Read the model definition and answer for the solid it produces. Units are mm, in the model's axes. A direction names the side the tool comes from. Give positions to 0.01 mm unless a question says otherwise; leave off trailing zeros. Order: outer loops, then holes, each group sorted by start corner. A loop starts at its lowest first (then second) coordinate and runs counter-clockwise, first axis right, second up. Notation, with made-up numbers: (18, 39.25) - (31, 39.25) arc R15 cw to (31, 52.25) - close; hole circle Ø2 at (15.5, -23). An arc over 180 degrees is marked (long way). Return JSON: item names as keys, results as strings.
```python
from build123d import *

# Parameters (mm, degrees)
BOSS_EXTRUDE1_DEPTH = 12.7
CUT_EXTRUDE2_DEPTH  = 4.5
CUT_EXTRUDE3_DEPTH  = 11.2
BOSS_EXTRUDE2_START = -7.7
SKETCH2_5_R         = 1.6
BOSS_EXTRUDE2_DEPTH = 9.1
SKETCH2_6_R         = 1.8
CUT_EXTRUDE4_DEPTH  = 11.2
SKETCH2_7_R         = 1.6
BOSS_EXTRUDE3_DEPTH = 1.4
SKETCH2_8_W         = 36
SKETCH2_8_H         = 0.65
CUT_EXTRUDE5_DEPTH  = 4
CUT_EXTRUDE6_DEPTH  = 3
SKETCH4_W           = 1.5
SKETCH4_H           = 22
CUT_EXTRUDE7_DEPTH  = 3
SKETCH6_W           = 2.1
SKETCH6_H           = 4.185
BOSS_EXTRUDE4_DEPTH = 1
CUT_EXTRUDE9_START  = -10.2
CUT_EXTRUDE9_DEPTH  = 4.5
FILLET3_R           = 1.5
FILLET2_R           = 0.25


with BuildPart() as part:
    # Sketch1 → Boss-Extrude1 (new body)
    with BuildSketch(Plane(origin=(0, 0, 0), x_dir=(1, 0, 0), z_dir=(0, 1, 0))):
        Polygon((-28.77817965, 9.54419618), (-24.27817965, 9.54419618), (-24.27817965, 17.54419618), (-21.57817965, 17.54419618), (-21.57817965, 9.54419618), (-18.57817965, 9.54419618), (-18.57817965, -18.45580382), (-21.07817965, -18.45580382), (-21.07817965, -4.45580382), (-28.77817965, -4.45580382), align=None)
    extrude(amount=BOSS_EXTRUDE1_DEPTH)

    # Sketch2 → Cut-Extrude2 (cut)
    with BuildSketch(Plane.ZY.offset(28.77817965)):
        Polygon((-9.54419618, 3.548072024), (-9.54419618, 0), (-3.657330191, 0), align=None)
    extrude(amount=-CUT_EXTRUDE2_DEPTH, mode=Mode.SUBTRACT)

    # Sketch2<4> → Cut-Extrude3 (cut, through all)
    with BuildSketch(Plane.ZY.offset(28.77817965)):
        Polygon((12.124702683, 0), (18.45580382, 0), (18.45580382, 9.2), align=None)
    extrude(amount=-CUT_EXTRUDE3_DEPTH, mode=Mode.SUBTRACT)

    # Sketch2<5> → Boss-Extrude2 (add)
    with BuildSketch(Plane.ZY.offset(28.77817965).offset(BOSS_EXTRUDE2_START)):
        with Locations((15.20580382, 9.2)):
            Circle(SKETCH2_5_R)
    extrude(amount=BOSS_EXTRUDE2_DEPTH)

    # Sketch2<6> → Cut-Extrude4 (cut, through all)
    with BuildSketch(Plane.ZY.offset(28.77817965)):
        with Locations((-13.54419618, 9.2)):
            Circle(SKETCH2_6_R)
    extrude(amount=-CUT_EXTRUDE4_DEPTH, mode=Mode.SUBTRACT)

    # Sketch2<7> → Boss-Extrude3 (add)
    with BuildSketch(Plane.ZY.offset(28.77817965)):
        with Locations((-6.29419618, 9.2)):
            Circle(SKETCH2_7_R)
    extrude(amount=BOSS_EXTRUDE3_DEPTH)

    # Sketch2<8> → Cut-Extrude5 (cut)
    with BuildSketch(Plane.ZY.offset(28.77817965)):
        with Locations((0.45580382, 11.625)):
            Rectangle(SKETCH2_8_W, SKETCH2_8_H)
    extrude(amount=-CUT_EXTRUDE5_DEPTH, mode=Mode.SUBTRACT)

    # Sketch3 → Cut-Extrude6 (cut)
    with BuildSketch(Plane(origin=(-18.57817965, 0, 0), x_dir=(0, 0, -1), z_dir=(1, 0, 0))):
        Polygon((9.54419618, 0), (9.54419618, 9.2), (-0.27080382, 0), align=None)
        Polygon((-12.124702683, 0), (-18.45580382, 9.2), (-18.45580382, 0), align=None)
        Polygon((-8.64080382, 0), (-18.45580382, 9.2), (-12.124702683, 0), align=None)
    extrude(amount=-CUT_EXTRUDE6_DEPTH, mode=Mode.SUBTRACT)

    # Sketch4 → Cut-Extrude7 (cut)
    with BuildSketch(Plane.XZ):
        with Locations((-22.92817965, -6.54419618)):
            Rectangle(SKETCH4_W, SKETCH4_H)
    extrude(amount=-CUT_EXTRUDE7_DEPTH, mode=Mode.SUBTRACT)

    # Sketch6 → Boss-Extrude4 (add)
    with BuildSketch(Plane(origin=(0, 0, 0), x_dir=(-1, 0, 0), z_dir=(0, -1, 0))):
        with Locations((22.62817965, -2.36330382)):
            Rectangle(SKETCH6_W, SKETCH6_H)
    extrude(amount=-BOSS_EXTRUDE4_DEPTH)

    # Sketch3<3> → Cut-Extrude9 (cut)
    with BuildSketch(Plane(origin=(-18.57817965, 0, 0), x_dir=(0, 0, -1), z_dir=(1, 0, 0)).offset(CUT_EXTRUDE9_START)):
        Polygon((9.54419618, 0), (9.54419618, 9.2), (-0.27080382, 0), align=None)
    extrude(amount=CUT_EXTRUDE9_DEPTH, mode=Mode.SUBTRACT)

    # Fillet3
    fillet3_edges = [part.edges().sort_by_distance(p)[0] for p in [
        (-18.57817965, 0, 4.45580382),
        (-18.57817965, 10.95, 18.45580382),
        (-18.57817965, 4.6, 13.54830382),
        (-18.57817965, 4.6, -4.63669618),
        (-18.57817965, 10.95, -9.54419618),
        (-18.57817965, 12.7, 4.45580382),
        (-24.92817965, 12.7, 4.45580382),
        (-19.82817965, 0, 8.64080382),
        (-19.82817965, 9.2, 18.45580382),
        (-19.82817965, 12.7, 18.45580382),
        (-26.52817965, 0, 0.27080382),
        (-20.07817965, 0, 0.27080382),
        (-20.07817965, 9.2, -9.54419618),
        (-20.07817965, 12.7, -9.54419618),
        (-26.52817965, 9.2, -9.54419618),
        (-26.52817965, 12.7, -9.54419618),
        (-21.87817965, 0, -17.54419618),
        (-23.97817965, 0, -17.54419618),
        (-22.92817965, 12.7, -17.54419618),
    ]]
    fillet(fillet3_edges, radius=FILLET3_R)

    # Fillet2
    fillet2_edges = [part.edges().sort_by_distance(p)[0] for p in [
        (-22.17817965, 3, -6.54419618),
        (-22.17817965, 2, 4.45580382),
        (-22.92817965, 3, -17.54419618),
        (-22.17817965, 2.25, -17.54419618),
        (-23.67817965, 3, -6.54419618),
        (-23.67817965, 2.25, -17.54419618),
        (-22.92817965, 3, 4.45580382),
        (-23.67817965, 2, 4.45580382),
        (-23.67817965, 0, -7.88669618),
        (-22.17817965, 0, -7.88669618),
        (-22.17817965, 0.439339828, -17.104856352),
        (-23.67817965, 0.439339828, -17.104856352),
    ]]
    fillet(fillet2_edges, radius=FILLET2_R)


solid = part.part
```
Q1. Given pin 1 (0.8 mm diameter, centred on y = 12, z = -1.5, fed in from -X); pin 2 (1.1 mm diameter, centred on x = -23.5, y = 0.5, fed in from -Z); pin 3 (0.7 mm diameter, centred on x = -27.5, y = 11, fed in from -Z), each flat-ended and moving along its own axis, determine where each tip first touches the part or whether it passes through.
Values:
{"pin 1": "stops at x = -28.78", "pin 2": "stops at z = -17.42", "pin 3": "stops at z = -9.54"}
Q2. Consider L1, parallel to X at y = 2, z = -4; L2, parallel to X at y = 10.75, z = 4; L3, parallel to X at y = 8.75, z = 12.5. Determine where each line is inside the solid, lowest interval first.
Values:
{"L1": "x = -24.28 to -23.68, -22.18 to -21.58", "L2": "x = -28.78 to -18.58", "L3": "x = -21.08 to -18.58"}
Q3. For faces 1 (the flat face through (-22.9, 0.5, 0.271)), 2 (the flat face through (-20.82, 4.64, -4.68)), 3 (the flat face through (-21, 11, -9.544)), 4 (the flat face through (-25, 6, 4.456)), 5 (the flat face through (-27, 11, -9.544)), determine the directions among +Z, -Z, +X, -X, +Y, -Y from which every point of the face is accessible in a straight line to the end or side of a thin tool.
Values:
{"face 1": "-Z, -Y", "face 2": "-Z, +X, -Y", "face 3": "-Z, +X, +Y, -Y", "face 4": "-X, +Y, -Y", "face 5": "-Z, -X, +Y, -Y"}
Q4. A cutting plane is placed at A-A (x = -23). Write down the section's boundary in (y, z), and give its area (3 significant figures).
Values:
{"outline": "(0, 0.27) - (1, 0.27) - (1, 4.46) - (0, 4.46) - close; (3, -17.29) arc R0.25 ccw to (3.25, -17.54) - (11.2, -17.54) arc R1.5 ccw to (12.7, -16.04) - (12.7, 2.96) arc R1.5 ccw to (11.2, 4.46) - (3.25, 4.46) arc R0.25 ccw to (3, 4.21) - close; circle Ø3.2 at (9.2, 15.21); hole circle Ø3.6 at (9.2, -13.54)", "area": "214 mm²"}
Q5. A cutting plane is placed at C-C (x = -19.5). Write down the section's boundary in (y, z), and give its area (3 significant figures).
Values:
{"outline": "(0.12, 0.86) arc R1.38 ccw to (0.49, -0.08) - (8.84, -8.99) arc R1.38 ccw to (9.85, -9.43) - (11.2, -9.43) arc R1.38 ccw to (12.58, -8.04) - (12.58, 16.96) arc R1.38 ccw to (11.2, 18.34) - (9.85, 18.34) arc R1.38 ccw to (8.84, 17.9) - (0.49, 8.99) arc R1.38 ccw to (0.12, 8.05) - close", "area": "256 mm²"}
Q6. Determine the mould class of faces 6 (the flat face through (-21.078, 8, 11)), 7 (the cylindrical face through (-19.03, 4.83, -4.26)), 8 (the flat face through (-22.178, 1, -7)) for opening direction Z: released by +Z, released by -Z, zero draft, split by the parting line, or undercut.
Values:
{"face 6": "undercut", "face 7": "released by -Z", "face 8": "zero draft"}
Q7. A cutting plane is placed at B-B (z = 7). Write down the section's boundary in (x, y), and give its area (3 significant figures).
Values:
{"outline": "(-21.08, 0) - (-20.08, 0) arc R1.5 ccw to (-18.58, 1.5) - (-18.58, 11.2) arc R1.5 ccw to (-20.08, 12.7) - (-21.08, 12.7) - close", "area": "30.8 mm²"}
